Input: part model. Units: mm. Frame: model coordinates. Face numbers are marked on the shaded views. A direction names the side the tool comes from. Give positions to 0.01 mm unless a question says otherwise; leave off trailing zeros. Order: outer loops, then holes, each group sorted by start corner. A loop starts at its lowest first (then second) coordinate and runs counter-clockwise, first axis right, second up. Notation, with made-up numbers: (50, 43) - (57, 43) arc R9 ccw to (57, 50) - close; hole circle Ø4 at (74.25, 6.25). An arc over 180 degrees is marked (long way). Answer in a Markdown table with one row per item. Add a question column.
1. Contact query for flat-ended pins moving along their axis: pin 1 (6 mm diameter, centred on y = 16, z = -107.5, fed in from -X); pin 2 (12 mm diameter, centred on x = -6.5, y = -7, fed in from +Z); pin 3 (3 mm diameter, centred on x = 13, y = -24.5, fed in from +Z). Output: stop coordinate, or through.
2. Ray query, line 1 (X direction, y = -0.5, z = -254.5); line 2 (Z direction, x = 3, y = 7); line 3 (Y direction, x = -1.5, z = -264.5). Return the intervals inside material, ascending. Write a range as [from, to].
3. Access query for the marked faces 1 and 2. Directions: +Z, -Z, +X, -X, +Y, -Y. A direction counts if a zero-diameter tool reaches every point of the face in a straight line with its end or side. Return the directions, or none.
4. Section query A-A on z = -147.5. Return loops of the section in (x, y), and give its area (3 significant figures).
```python
from build123d import *

# Parameters (mm, degrees)
FILLET1_R = 12.7
FILLET2_R = 6.35


with BuildPart() as part:
    # Sketch1 → Revolve1 (revolve)
    with BuildSketch(Plane(origin=(0, 0, 0), x_dir=(0, 0, -1), z_dir=(1, 0, 0))):
        Polygon((0, 0), (0, 3.175), (1.27, 3.175), (1.27, 14.732), (9.398, 14.732), (9.398, 32.512), (275.082, 32.512), (275.082, 35.306), (283.972, 35.306), (288.544, 32.555084127), (299.466, 14.732), (307.594, 14.732), (307.594, 3.175), (308.864, 3.175), (308.864, 0), align=None)
    revolve(axis=Axis((0, 0, 0), (0, 0, -1)))

    # Fillet1
    fillet1_edges = [part.edges().sort_by_distance(p)[0] for p in [
        (0, -32.512, -9.398),
    ]]
    fillet(fillet1_edges, radius=FILLET1_R)

    # Fillet2
    fillet2_edges = [part.edges().sort_by_distance(p)[0] for p in [
        (0, -35.306, -283.972),
    ]]
    fillet(fillet2_edges, radius=FILLET2_R)


solid = part.part
```
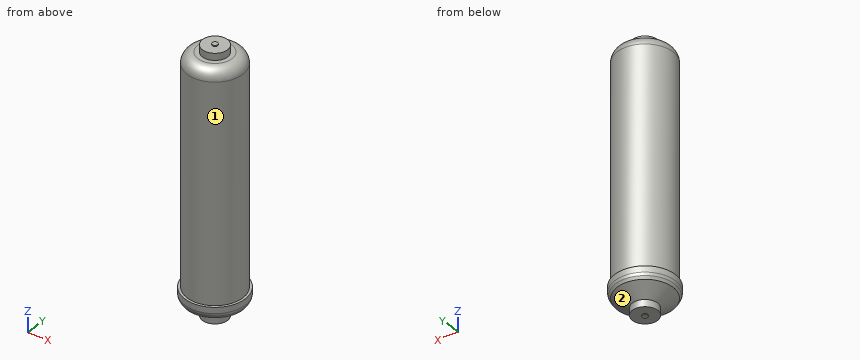
Answer:
| question | item | result |
|---|---|---|
| 1 | pin 1 | stops at x = -29.8 |
| 1 | pin 2 | stops at z = -1.27 |
| 1 | pin 3 | stops at z = -11.14 |
| 2 | line 1 | x = [-32.51, 32.51] |
| 2 | line 2 | z = [-307.59, -1.27] |
| 2 | line 3 | y = [-32.48, 32.48] |
| 3 | face 1 | +Z |
| 3 | face 2 | -Z |
| 4 | outline | circle Ø65.02 at (0, 0) |
| 4 | area | 3,320 mm² |
